Source: three-view drawing plus pictorial views. Frame: mm from the lowest corner of the part. A direction names the side the tool comes from. Round coordinates to 2 decimals unless told otherwise and drop trailing zeros. Loops run counter-clockwise (first coordinate to the right, second up) from the corner with the lowest first, then second, coordinate; pieces in that order, holes last. Notation, with made-up numbers: (51, -25) -> (93, -25) arc R25 ccw to (93, 7) -> close; hole circle Ø4 at (0.5, -20.5). An arc over 180 degrees is marked (long way). Answer in a Markdown table with one row per item. Add a question column.
Q1. Section D-D, the plane z = 0.3. Output: boundary loops of the cut face in (x, y).
Q2. Ray query, L1, parallel to Y at x = 5.5, z = 1.2; L2, parallel to X at y = 1.5, z = 1.5; L3, parallel to X at y = 3, z = 2. Return the intervals inside material, ascending. Write a range as from..to.
Q3. Section B-B, the plane y = 5. Output: boundary loops of the cut face in (x, z), and give its area (3 significant figures).
Q4. Pin query (flat end, axial travel): pin 1 (0.6 mm diameter, centred on x = 4.5, z = 2, fed in from +Y); pin 2 (1 mm diameter, centred on y = 5, z = 2, fed in from +X); pin 3 (0.5 mm diameter, centred on x = 5, y = 8.5, fed in from +Z); pin 4 (1.5 mm diameter, centred on x = 8, y = 5, fed in from +Z). Return the tip coordinate at first contact, or that it passes through.
Q5. Reachability of the marked faces 1, 2, 3 and 4 from +Z, -Z, +X, -X, +Y, -Y: full face, straight path, thin tool, end or side. Return the list, or none.
Q6. Section A-A, the plane z = 1.5. Output: boundary loops of the cut face in (x, y), and give its area (3 significant figures).
Q7. Mould query, pull axis Y, two halves, no side actions, for the marked faces 5, 6 and 7. Classes: pulls with the +Y half, pulls with the -Y half, needs draft (parallel to the pull), parting line crosses it, or undercut.
Q8. Section C-C, the plane x = 5. Output: boundary loops of the cut face in (y, z), and give its area (3 significant figures).
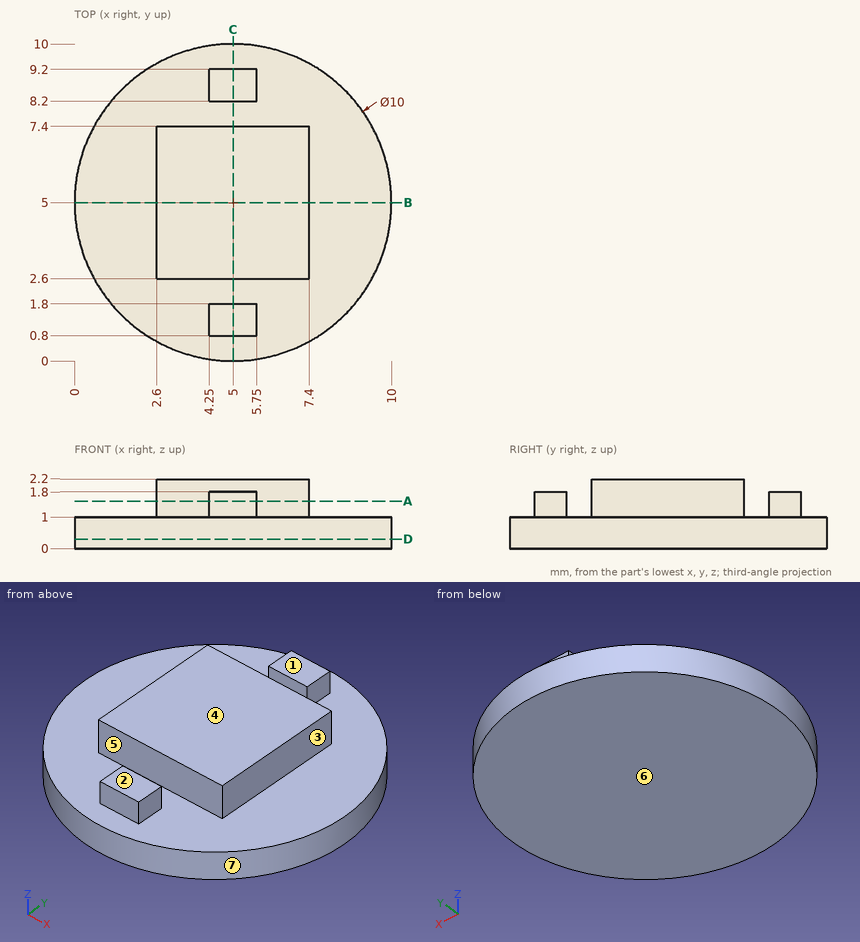
Answer block:
| question | item | result |
|---|---|---|
| 1 | outline | circle Ø10 at (5, 5) |
| 2 | L1 | 0.8..1.8, 2.6..7.4, 8.2..9.2 |
| 2 | L2 | 4.25..5.75 |
| 2 | L3 | 2.6..7.4 |
| 3 | outline | (0, 0) -> (10, 0) -> (10, 1) -> (7.4, 1) -> (7.4, 2.2) -> (2.6, 2.2) -> (2.6, 1) -> (0, 1) -> close |
| 3 | area | 15.8 mm^2 |
| 4 | pin 1 | y = 9.2 |
| 4 | pin 2 | x = 7.4 |
| 4 | pin 3 | z = 1.8 |
| 4 | pin 4 | z = 2.2 |
| 5 | face 1 | +Z, +X, -X, +Y |
| 5 | face 2 | +Z, +X, -X, -Y |
| 5 | face 3 | +Z, +X, +Y, -Y |
| 5 | face 4 | +Z, +X, -X, +Y, -Y |
| 6 | outline | (2.6, 2.6) -> (7.4, 2.6) -> (7.4, 7.4) -> (2.6, 7.4) -> close; (4.25, 0.8) -> (5.75, 0.8) -> (5.75, 1.8) -> (4.25, 1.8) -> close; (4.25, 8.2) -> (5.75, 8.2) -> (5.75, 9.2) -> (4.25, 9.2) -> close |
| 6 | area | 26.0 mm^2 |
| 7 | face 5 | undercut |
| 7 | face 6 | needs draft |
| 7 | face 7 | parting line crosses it |
| 8 | outline | (0, 0) -> (10, 0) -> (10, 1) -> (9.2, 1) -> (9.2, 1.8) -> (8.2, 1.8) -> (8.2, 1) -> (7.4, 1) -> (7.4, 2.2) -> (2.6, 2.2) -> (2.6, 1) -> (1.8, 1) -> (1.8, 1.8) -> (0.8, 1.8) -> (0.8, 1) -> (0, 1) -> close |
| 8 | area | 17.4 mm^2 |
